```python
from build123d import *

# Parameters (mm, degrees)
SKETCH1_W           = 15
SKETCH1_H           = 10
SKETCH1_H_2         = 15
SKETCH1_W_2         = 10
BOSS_EXTRUDE1_DEPTH = 16.7
SKETCH2_R           = 6.5
CUT_EXTRUDE1_DEPTH  = 8.3
SKETCH3_R           = 6.5
CUT_EXTRUDE2_DEPTH  = 8.3
SKETCH4_R           = 6.5
CUT_EXTRUDE3_DEPTH  = 14.7
SKETCH5_W           = 42
SKETCH5_H           = 42
SKETCH5_R           = 2.6
BOSS_EXTRUDE3_DEPTH = 16.7
FILLET9_SIZE        = 2
BOSS_EXTRUDE4_START = 32
SKETCH7_R           = 6.5
BOSS_EXTRUDE4_DEPTH = 32
BOSS_EXTRUDE5_START = 32
SKETCH8_R           = 6.5
BOSS_EXTRUDE5_DEPTH = 32
CUT_EXTRUDE4_DEPTH  = 5
CHAMFER1_SIZE       = 2


with BuildPart() as part:
    # Sketch1 → Boss-Extrude1 (new body)
    with BuildSketch(Plane(origin=(0, 0, 0), x_dir=(1, 0, 0), z_dir=(0, 1, 0))):
        Rectangle(SKETCH1_W, SKETCH1_H)
        with Locations((0, 12.5)):
            Rectangle(SKETCH1_W, SKETCH1_H_2)
        with Locations((12.5, 12.5)):
            Rectangle(SKETCH1_W_2, SKETCH1_H_2)
    extrude(amount=BOSS_EXTRUDE1_DEPTH)

    # Sketch2 → Cut-Extrude1 (cut)
    with BuildSketch(Plane.XY.offset(5)):
        with Locations((0, 8.35)):
            Circle(SKETCH2_R)
    extrude(amount=-CUT_EXTRUDE1_DEPTH, mode=Mode.SUBTRACT)

    # Sketch3 → Cut-Extrude2 (cut)
    with BuildSketch(Plane(origin=(17.5, 0, 0), x_dir=(0, 0, -1), z_dir=(1, 0, 0))):
        with Locations((12.5, 8.35)):
            Circle(SKETCH3_R)
    extrude(amount=-CUT_EXTRUDE2_DEPTH, mode=Mode.SUBTRACT)

    # Sketch4 → Cut-Extrude3 (cut)
    with BuildSketch(Plane.XZ):
        with Locations(Location((0, -12.5, 0), (0, 0, 270))):
            Circle(SKETCH4_R)
    extrude(amount=-CUT_EXTRUDE3_DEPTH, mode=Mode.SUBTRACT)

    # Fillet8
    # the kernel refuses this chamfer: 2 mm, written as the material it takes off along each edge
    with BuildSketch(Plane(origin=(-6.166666667, 1.333333333, -18.666666667), x_dir=(0.7071067811865471, 0, -0.707106781186548), z_dir=(-0.5773502691896263, -0.5773502691896255, -0.5773502691896254)), Plane(origin=(-6.166666667, 15.366666667, -18.666666667), x_dir=(0.7071067811865471, 0.7071067811865478, 0), z_dir=(-0.5773502691896261, 0.5773502691896256, -0.5773502691896256))) as fillet8_piece_1:
        Polygon((-1.414213562, -0.816496581), (1.414213562, -0.816496581), (0, 1.632993162), align=None)
    extrude(amount=2.540341184, mode=Mode.SUBTRACT)
    with BuildSketch(Plane(origin=(-7.5, 0, -25.143365976), x_dir=(-0.027495876610586494, 0.9996219169112968, 0), z_dir=(0, 0, 1)), Plane(origin=(22.643365976, 16.7, -20), x_dir=(0, 0.027495876610585647, 0.9996219169112968), z_dir=(-1, 0, 0)), Plane(origin=(-7.5, 16.7, 10.143365976), x_dir=(-0.027495876610586487, -0.9996219169112968, 0), z_dir=(0, 0, -1)), Plane(origin=(22.643365976, 0, -20), x_dir=(0, 0.9996219169112968, -0.02749587661058563), z_dir=(-1, 0, 0))) as fillet8_piece_2:
        with BuildLine():
            Line((2.05734639, 0), (-0.11309431, -2.054235587))
            Line((-0.11309431, -2.054235587), (-0.153079186, -2.053135752))
            ThreePointArc((-0.153079186, -2.053135752), (-0.068258454, -1.026795659), (-0.039984877, 0.001099835))
            Line((-0.039984877, 0.001099835), (0.001099835, 0.039984877))
            ThreePointArc((0.001099835, 0.039984877), (1.028995329, 0.011711299), (2.058446225, 0.039984877))
            Line((2.058446225, 0.039984877), (2.05734639, 0))
        make_face()
    extrude(amount=35.286731952, mode=Mode.SUBTRACT)
    with BuildSketch(Plane(origin=(-7.5, -5.143365976, -20), x_dir=(-0.02749587661058694, 0, 0.9996219169112968), z_dir=(0, 1, 0))) as fillet8_piece_3:
        with BuildLine():
            Line((2.05734639, 0), (-0.11309431, 2.054235587))
            Line((-0.11309431, 2.054235587), (-0.153079186, 2.053135752))
            ThreePointArc((-0.153079186, 2.053135752), (-0.068258454, 1.026795659), (-0.039984877, -0.001099835))
            Line((-0.039984877, -0.001099835), (0.001099835, -0.039984877))
            ThreePointArc((0.001099835, -0.039984877), (1.028995329, -0.011711299), (2.058446225, -0.039984877))
            Line((2.058446225, -0.039984877), (2.05734639, 0))
        make_face()
    extrude(amount=26.986731952, mode=Mode.SUBTRACT)

    # Sketch5 → Boss-Extrude3 (add)
    with BuildSketch(Plane(origin=(0, 16.7, 0), x_dir=(1, 0, 0), z_dir=(0, 1, 0))):
        with Locations((28.5, -16)):
            Rectangle(SKETCH5_W, SKETCH5_H)
        with Locations(Location((28.5, -16, 0), (0, 0, 270))):
            Circle(SKETCH5_R, mode=Mode.SUBTRACT)
    extrude(amount=-BOSS_EXTRUDE3_DEPTH)

    # Fillet9
    fillet9_edges = [part.edges().sort_by_distance(p)[0] for p in [
        (49.5, 8.35, 37),
    ]]
    chamfer(fillet9_edges, length=FILLET9_SIZE)

    # Sketch7 → Boss-Extrude4 (add)
    with BuildSketch(Plane.XY.offset(5).offset(BOSS_EXTRUDE4_START)):
        Polygon((-5.5, 16.7), (-7.5, 14.7), (-7.5, 2), (-5.5, 0), (7.5, 0), (7.5, 16.7), align=None)
        with Locations((0, 8.35)):
            Circle(SKETCH7_R, mode=Mode.SUBTRACT)
    extrude(amount=-BOSS_EXTRUDE4_DEPTH)

    # Sketch8 → Boss-Extrude5 (add)
    with BuildSketch(Plane(origin=(17.5, 0, 0), x_dir=(0, 0, -1), z_dir=(1, 0, 0)).offset(BOSS_EXTRUDE5_START)):
        Polygon((5, 16.7), (5, 0), (18, 0), (20, 2), (20, 14.7), (18, 16.7), align=None)
        with Locations((12.5, 8.35)):
            Circle(SKETCH8_R, mode=Mode.SUBTRACT)
    extrude(amount=-BOSS_EXTRUDE5_DEPTH)

    # Sketch9 → Cut-Extrude4 (cut)
    with BuildSketch(Plane.XZ):
        with BuildLine():
            Line((28.5, 8.5), (49.5, 8.5))
            Line((49.5, 8.5), (49.5, 35))
            Line((49.5, 35), (47.5, 37))
            Line((47.5, 37), (28.5, 37))
            Line((28.5, 37), (21, 37))
            Line((21, 37), (21, 16))
            ThreePointArc((21, 16), (23.196699141, 10.696699141), (28.5, 8.5))
        make_face()
    extrude(amount=-CUT_EXTRUDE4_DEPTH, mode=Mode.SUBTRACT)

    # Chamfer1
    # the kernel refuses this chamfer: 2 mm, written as the material it takes off along each edge
    with BuildSketch(Plane(origin=(49.5, 16.7, 40.143365976), x_dir=(-0.9996219169112968, 0.027495876610585647, 0), z_dir=(0, 0, -1)), Plane(origin=(-10.643365976, 16.7, 37), x_dir=(0, 0.027495876610585647, -0.9996219169112968), z_dir=(1, 0, 0))) as chamfer1_piece_1:
        Polygon((CHAMFER1_SIZE * 0.999621916911, -CHAMFER1_SIZE * 0.0274958766106), (-CHAMFER1_SIZE * 0.0274958766106, -CHAMFER1_SIZE * 0.999621916911), (0, 0), align=None)
    extrude(amount=63.286731952, mode=Mode.SUBTRACT)


solid = part.part
```
Design review of the part built by this model. Coordinates are the model's own, in mm. A direction names the side the tool comes from. Coordinates: 2 decimals unless noted, no trailing zeros. Order: outer loops, then holes, each group sorted by start corner. A loop starts at its lowest first (then second) coordinate and runs counter-clockwise, first axis right, second up. Notation, with made-up numbers: (-21.5, -23) - (7.5, -23) arc R7 cw to (7.5, -12) - close; hole circle Ø2 at (66.25, -35.5). An arc over 180 degrees is marked (long way). Answer in a Markdown table with one row per item.
(1) The part is to be moulded in two halves that separate along Y. For faces 1 (the cylindrical face through (-0.8, 14.8, 17.1)), 2 (the flat face through (48.5, 15.7, 8.4)), 3 (the cylindrical face through (23.139, 2.465, 10.755)), say which applies: released by +Y, released by -Y, zero draft, split by the parting line, or undercut.
Checked values:
| item | result |
|---|---|
| face 1 | undercut |
| face 2 | released by +Y |
| face 3 | zero draft |
(2) Consider section A-A on z = 32. State the section outline as (x, y) points.
Checked values:
| item | result |
|---|---|
| outline | (-7.5, 2) - (-5.5, 0) - (21, 0) - (21, 5) - (49.5, 5) - (49.5, 14.7) - (47.5, 16.7) - (-5.5, 16.7) - (-7.5, 14.7) - close; hole circle Ø13 at (0, 8.35) |
(3) Clearance check with a flat-ended pin moving along its axis: pin 1 (4 mm diameter, centred on x = 43.5, y = 2, fed in from +Z). State where the tip first meets the part, or that it passes through.
Checked values:
| item | result |
|---|---|
| pin 1 | z = 8.5 |
(4) Consider section C-C on x = 40. State the section outline as (y, z) points.
Checked values:
| item | result |
|---|---|
| outline | (0, -18) - (2, -20) - (14.7, -20) - (16.7, -18) - (16.7, 35) - (14.7, 37) - (5, 37) - (5, 8.5) - (0, 8.5) - close; hole circle Ø13 at (8.35, -12.5) |
(5) Consider section B-B on x = 27. State the section outline as (y, z) points, plus the area to 3 significant figures.
Checked values:
| item | result |
|---|---|
| outline | (0, -18) - (2, -20) - (14.7, -20) - (16.7, -18) - (16.7, 13.88) - (5, 13.88) - (5, 8.65) - (0, 8.65) - close; (5, 18.12) - (16.7, 18.12) - (16.7, 35) - (14.7, 37) - (5, 37) - close; hole circle Ø13 at (8.35, -12.5) |
| area | 622 mm^2 |
(6) For faces 4 (the cylindrical face through (5.481, 7.247, -15.994)), 5 (the flat face through (49.5, 9, 8)), 6 (the flat face through (0, 8, -3.3)), 7 (the flat face through (9.2, 8, -12)), 8 (the flat face through (21, 2, 27)), list the 3-axis set-ups (+Z, -Z, +X, -X, +Y, -Y) from which the entire face can be reached by the end or side of a thin tool; tool diameter is ignored.
Checked values:
| item | result |
|---|---|
| face 4 | -Y |
| face 5 | +Z, -Z, +X, +Y, -Y |
| face 6 | +Z |
| face 7 | +X |
| face 8 | +Z, +X, -Y |
(7) Wall thickness on line 1 along Z through (x, y) = (0, 11.25); line 2 along X through (y, z) = (7, 14); line 3 along X through (y, z) = (12.75, 15): over which ranges is each line inside the solid? List them lowest first. Write a range as from..to.
Checked values:
| item | result |
|---|---|
| line 1 | -20..-19, -6..-3.3 |
| line 2 | -7.5..-6.36, 6.36..26.84, 30.16..49.5 |
| line 3 | -7.5..-4.78, 4.78..26.1, 30.9..49.5 |
(8) Consider section D-D on y = 6. State the section outline as (x, z) points, plus the area to 3 significant figures.
Checked values:
| item | result |
|---|---|
| outline | (-7.5, -18) - (-5.5, -20) - (49.5, -20) - (49.5, -18.56) - (9.2, -18.56) - (9.2, -6.44) - (49.5, -6.44) - (49.5, 35) - (47.5, 37) - (6.06, 37) - (6.06, -3.3) - (-6.06, -3.3) - (-6.06, 37) - (-7.5, 37) - close; hole circle Ø13 at (0, -12.5); hole circle Ø5.2 at (28.5, 16) |
| area | 2,110 mm^2 |
